Geometry: final body of the model. Coordinates: model frame, mm. A direction names the side the tool comes from. Give positions to 0.01 mm unless a question says otherwise; leave off trailing zeros. Write each loop counter-clockwise with the first axis right and the second up, starting at its lowest first coordinate (ties: lowest second). Pieces come first, ordered by that corner, then holes. Notation, with made-up numbers: M 58.5,32.25 L 81.5,32.25 A27 ccw 81.5,71.25 Z; hole C 83,7 d2. An arc over 180 degrees is marked long. Answer as a JSON object with one key per item and string values.
from build123d import *

# Parameters (mm, degrees)
F1_DEPTH = 3.81


# Not quite as in the source:
# - a feature names something its author has since deleted; it is built from what else it names


with BuildPart() as f1:
    # F0 (on Front) → F1 (new body)
    with BuildSketch(Plane.XZ):
        Polygon((89, 20.5917087717), (89, 27.203), (82.18, 27.203), (64, 27.203), (54, 27.203), (39, 27.203), (0, 27.203), (0, 0), (89, 0), (89, 5.5917087717), (85.19, 5.5917087717), (85.19, 20.5917087717), align=None)
        Polygon((-89, 0), (0, 0), (0, 27.203), (-39, 27.203), (-54, 27.203), (-64, 27.203), (-82.18, 27.203), (-89, 27.203), (-89, 20.5917087717), (-85.19, 20.5917087717), (-85.19, 5.5917087717), (-89, 5.5917087717), align=None)
        Polygon((0, -27.203), (0, 0), (-89, 0), (-89, -4.6252912283), (-85.19, -4.6252912283), (-85.19, -19.6252912283), (-89, -19.6252912283), (-89, -27.203), (-82.18, -27.203), (-64, -27.203), (-54, -27.203), (-39, -27.203), align=None)
        Polygon((89, -4.6252912283), (89, 0), (0, 0), (0, -27.203), (39, -27.203), (54, -27.203), (64, -27.203), (82.18, -27.203), (89, -27.203), (89, -19.6252912283), (85.19, -19.6252912283), (85.19, -4.6252912283), align=None)
    extrude(amount=F1_DEPTH)


solid = f1.part
1) Contact query for flat-ended pins moving along their axis: P1, Ø2, axis at x = -55, z = 14, coming from the +Y side; P2, Ø1.1, axis at y = -3, z = 12, coming from the +X side. Output: stop coordinate, or through.
Geometry check:
{"P1": "stops at y = 0", "P2": "stops at x = 85.19"}
2) Line query: line 1 (X direction, y = -0.8, z = -12.5). Output: solid intervals per line, ascending. Write a range as from..to.
Geometry check:
{"line 1": "x = -85.19..85.19"}
3) Pull-direction query (Z, two-part tool) for faces 4 (the flat face through (85.19, -2, 13)), 5 (the flat face through (-89, -2, 24)), 6 (the flat face through (1, -2, 27.203)), 7 (the flat face through (-1, -2, -27.203)); classes: pulls with the +Z half, pulls with the -Z half, needs draft (parallel to the pull), parting line crosses it, or undercut.
Geometry check:
{"face 4": "undercut", "face 5": "needs draft", "face 6": "pulls with the +Z half", "face 7": "pulls with the -Z half"}
4) Cut plane A-A on y = -0.65. Return loops of the section in (x, z), and give its area (3 significant figures).
Geometry check:
{"outline": "M -89,-27.2 L 89,-27.2 L 89,-19.63 L 85.19,-19.63 L 85.19,-4.63 L 89,-4.63 L 89,5.59 L 85.19,5.59 L 85.19,20.59 L 89,20.59 L 89,27.2 L -89,27.2 L -89,20.59 L -85.19,20.59 L -85.19,5.59 L -89,5.59 L -89,-4.63 L -85.19,-4.63 L -85.19,-19.63 L -89,-19.63 Z", "area": "9,460 mm2"}
5) Cut plane B-B on z = -16. Return loops of the section in (x, y), and give its area (3 significant figures).
Geometry check:
{"outline": "M -85.19,-3.81 L 85.19,-3.81 L 85.19,0 L -85.19,0 Z", "area": "649 mm2"}
6) Set-up query: faces 1 (the flat face through (89, -2, 0)), 2 (the flat face through (-85.19, -2, -12)), 3 (the flat face through (87, -2, -19.625)). Return all of +Z, -Z, +X, -X, +Y, -Y with unobstructed straight access to the full face (end or side cutting, diameter ignored); none if empty.
Geometry check:
{"face 1": "+Z, -Z, +X, +Y, -Y", "face 2": "-X, +Y, -Y", "face 3": "+X, +Y, -Y"}
